The listing builds one solid part. Answer for the finished solid, in the listing's coordinates (mm). A direction names the side the tool comes from. Give positions to 0.01 mm unless a question says otherwise; leave off trailing zeros. Loops run counter-clockwise (first coordinate to the right, second up) from the corner with the lowest first, then second, coordinate; pieces in that order, holes last. Notation, with made-up numbers: (56.25, 37) - (112.25, 37) arc R25 ccw to (112.25, 71) - close; hole circle Ø3 at (-20, -18.75). An arc over 180 degrees is marked (long way). One line per item, written item: value. Start each with the question number.
from build123d import *

# Parameters (mm, degrees)
F0_W     = 63.5
F0_H     = 50.8
F0_R     = 2.54
F2_DEPTH = 6.35
F1_W     = 63.5
F1_H     = 38.1
F1_R     = 3.81
F3_DEPTH = 6.35


with BuildPart() as f2:
    # F0 (on Top) → F2 (new body)
    with BuildSketch(Plane.XY):
        with Locations((2.81966, -11.114502)):
            Rectangle(F0_W, F0_H)
        with Locations((-12.351194, -16.165679)):
            Circle(F0_R, mode=Mode.SUBTRACT)
        with Locations((14.480258, -16.165679)):
            Circle(F0_R, mode=Mode.SUBTRACT)
    extrude(amount=F2_DEPTH)

    # F1 (on Front) → F3 (join)
    with BuildSketch(Plane.XZ):
        with Locations((2.38584, -19.05)):
            Rectangle(F1_W, F1_H)
        with Locations((0, -28.760821)):
            Circle(F1_R, mode=Mode.SUBTRACT)
        with Locations((0, -9.743084)):
            Circle(F1_R, mode=Mode.SUBTRACT)
    extrude(amount=F3_DEPTH)


solid = f2.part
1. A cutting plane is placed at C-C (x = 0). Determine the outline of the cut face in (y, z).
2. A cutting plane is placed at B-B (z = -26.5). Determine the outline of the cut face in (x, y), plus the area to 3 significant figures.
3. Find the intervals of material crossed by L1, parallel to Z at x = 0, y = -2; L2, parallel to X at y = -3.5, z = -9.5; L3, parallel to Z at x = 14, y = -29.5, in increasing order. Write a range as [from, to].
4. A cutting plane is placed at D-D (z = 3.5). Determine the outline of the cut face in (x, y).
5. A cutting plane is placed at A-A (x = 7). Determine the outline of the cut face in (y, z).
6. For faces 4 (the flat face through (2, 0, -19)), 5 (the flat face through (-28.93, -11, 3)), 6 (the flat face through (34.57, -11, 3)), determine the directions among +Z, -Z, +X, -X, +Y, -Y from which every point of the face is accessible in a straight line to the end or side of a thin tool.
7. Flat-ended cylindrical pins translate along their axes: pin 1 (1.5 mm diameter, centred on x = -7, y = -30, fed in from -Z); pin 2 (4.5 mm diameter, centred on x = 0, z = -9.74, fed in from +Y); pin 3 (6 mm diameter, centred on y = 1.5, z = -23, fed in from +X); pin 4 (5 mm diameter, centred on x = 22.5, z = -32.5, fed in from -Y). Find the tip coordinate at first contact, or state that the pin passes through.
8. Determine the mould class of faces 1 (the cylindrical face through (16.903, -15.403, 3.131)), 2 (the flat face through (2, -6.35, -19)), 3 (the flat face through (34.136, -3, -19)) for opening direction X: released by +X, released by -X, zero draft, split by the parting line, or undercut.
Results below:
1. outline: (-36.51, 0) - (-6.35, 0) - (-6.35, -5.93) - (0, -5.93) - (0, 0) - (14.29, 0) - (14.29, 6.35) - (-36.51, 6.35) - close; (-6.35, -38.1) - (0, -38.1) - (0, -32.57) - (-6.35, -32.57) - close; (-6.35, -24.95) - (0, -24.95) - (0, -13.55) - (-6.35, -13.55) - close
2. outline: (-29.36, -6.35) - (-3.07, -6.35) - (-3.07, 0) - (-29.36, 0) - close; (3.07, -6.35) - (34.14, -6.35) - (34.14, 0) - (3.07, 0) - close
2. area: 364 mm^2
3. L1: z = [-38.1, -32.57], [-24.95, -13.55], [-5.93, 6.35]
3. L2: x = [-29.36, -3.8], [3.8, 34.14]
3. L3: z = [0, 6.35]
4. outline: (-28.93, -36.51) - (34.57, -36.51) - (34.57, 14.29) - (-28.93, 14.29) - close; hole circle Ø5.08 at (-12.35, -16.17); hole circle Ø5.08 at (14.48, -16.17)
5. outline: (-36.51, 0) - (-6.35, 0) - (-6.35, -38.1) - (0, -38.1) - (0, 0) - (14.29, 0) - (14.29, 6.35) - (-36.51, 6.35) - close
6. face 4: -Z, +X, -X, +Y
6. face 5: +Z, -X, +Y, -Y
6. face 6: +Z, -Z, +X, +Y, -Y
7. pin 1: stops at z = 0
7. pin 2: passes through
7. pin 3: stops at x = 34.14
7. pin 4: stops at y = -6.35
8. face 1: undercut
8. face 2: zero draft
8. face 3: released by +X
